from build123d import *

# Parameters (mm, degrees)
SKIZZE1_W                       = 100
SKIZZE1_H                       = 30
AUFSATZ_LINEAR_AUSTRAGEN1_DEPTH = 6
DURCHGANGSLOCH_F_R_M31_DEPTH    = 6
DURCHGANGSLOCH_F_R_M32_DEPTH    = 6
M3_GEWINDEBOHRUNG1_D            = 2.5
SKIZZE12_W                      = 12
SKIZZE12_H                      = 4
SCHNITT_LINEAR_AUSTRAGEN1_DEPTH = 25
VERRUNDUNG1_R                   = 2.5
SKIZZE13_W                      = 10
SKIZZE13_H                      = 30
SCHNITT_LINEAR_AUSTRAGEN2_DEPTH = 1.5
F_2_0MM_STIFTLOCH1_D            = 2
F_2_0MM_STIFTLOCH1_DEPTH        = 8.5
F_2_0MM_STIFTLOCH1_TIP          = 0.600860619


# Read off the part's stored shape, not the designer's step: Durchgangsloch für M31, Durchgangsloch für M32
with BuildPart() as part:
    # Skizze1 → Aufsatz-Linear austragen1 (new body)
    with BuildSketch(Plane(origin=(0, 0, 0), x_dir=(1, 0, 0), z_dir=(0, 1, 0))):
        Rectangle(SKIZZE1_W, SKIZZE1_H)
    extrude(amount=AUFSATZ_LINEAR_AUSTRAGEN1_DEPTH)

    # Durchgangsloch für M31 outline → Durchgangsloch für M31 (cut)
    with BuildSketch(Plane(origin=(0, 0, 0), x_dir=(1, 0, 0), z_dir=(0, 1, 0))):
        with BuildLine():
            Line((-43.4, -9.6), (23.4, -9.6))
            ThreePointArc((23.4, -9.6), (25, -8), (23.4, -6.4))
            Line((23.4, -6.4), (-43.4, -6.4))
            ThreePointArc((-43.4, -6.4), (-45, -8), (-43.4, -9.6))
        make_face()
        with BuildLine():
            Line((-43.4, 6.4), (23.4, 6.4))
            ThreePointArc((23.4, 6.4), (25, 8), (23.4, 9.6))
            Line((23.4, 9.6), (-43.4, 9.6))
            ThreePointArc((-43.4, 9.6), (-45, 8), (-43.4, 6.4))
        make_face()
    extrude(amount=DURCHGANGSLOCH_F_R_M31_DEPTH, mode=Mode.SUBTRACT)

    # Durchgangsloch für M32 outline → Durchgangsloch für M32 (cut)
    with BuildSketch(Plane(origin=(0, 0, 0), x_dir=(1, 0, 0), z_dir=(0, 1, 0))):
        with BuildLine():
            ThreePointArc((46.6, 10.605062793), (45, 12.205062793), (43.4, 10.605062793))
            Line((43.4, 10.605062793), (43.4, 3.805062793))
            ThreePointArc((43.4, 3.805062793), (45, 2.205062793), (46.6, 3.805062793))
            Line((46.6, 3.805062793), (46.6, 10.605062793))
        make_face()
        with BuildLine():
            Line((46.6, -10.605062793), (46.6, -3.805062793))
            ThreePointArc((46.6, -3.805062793), (45, -2.205062793), (43.4, -3.805062793))
            Line((43.4, -3.805062793), (43.4, -10.605062793))
            ThreePointArc((43.4, -10.605062793), (45, -12.205062793), (46.6, -10.605062793))
        make_face()
    extrude(amount=DURCHGANGSLOCH_F_R_M32_DEPTH, mode=Mode.SUBTRACT)

    # M3 Gewindebohrung1 (through all)
    with Locations(Plane(origin=(0, 6, 0), x_dir=(1, 0, 0), z_dir=(0, 1, 0))):
        with Locations((-40, 0), (-20, 0)):
            Hole(M3_GEWINDEBOHRUNG1_D / 2)

    # Skizze12 → Schnitt-Linear austragen1 (cut)
    with BuildSketch(Plane.ZY.offset(50)):
        with Locations((9, 2)):
            Rectangle(SKIZZE12_W, SKIZZE12_H)
    extrude(amount=-SCHNITT_LINEAR_AUSTRAGEN1_DEPTH, mode=Mode.SUBTRACT)

    # Verrundung1
    verrundung1_edges = [part.edges().sort_by_distance(p)[0] for p in [
        (-25, 2, 3),
    ]]
    fillet(verrundung1_edges, radius=VERRUNDUNG1_R)

    # Skizze13 → Schnitt-Linear austragen2 (cut)
    with BuildSketch(Plane(origin=(0, 6, 0), x_dir=(1, 0, 0), z_dir=(0, 1, 0))):
        with Locations((45, 0)):
            Rectangle(SKIZZE13_W, SKIZZE13_H)
    extrude(amount=-SCHNITT_LINEAR_AUSTRAGEN2_DEPTH, mode=Mode.SUBTRACT)

    # Ø2.0mm Stiftloch1
    with Locations(Plane(origin=(0, 4.5, 0), x_dir=(1, 0, 0), z_dir=(0, 1, 0))):
        with Locations((45, 0)):
            Hole(F_2_0MM_STIFTLOCH1_D / 2, depth=F_2_0MM_STIFTLOCH1_DEPTH)
            with Locations((0, 0, -(F_2_0MM_STIFTLOCH1_DEPTH + F_2_0MM_STIFTLOCH1_TIP / 2))):  # 118° drill point
                Cone(0, F_2_0MM_STIFTLOCH1_D / 2, F_2_0MM_STIFTLOCH1_TIP, mode=Mode.SUBTRACT)


solid = part.part
Read the model definition and answer for the solid it produces. Units are mm, in the model's axes. A direction names the side the tool comes from. Round coordinates to 2 decimals unless told otherwise and drop trailing zeros. Write each loop counter-clockwise with the first axis right and the second up, starting at its lowest first coordinate (ties: lowest second). Pieces come first, ordered by that corner, then holes.
1. The part is cut by section B-B, the plane x = 45. Determine the outline of the cut face in (y, z), then the cut area to 3 significant figures.
2. Straight lines are drawn through the part: L1, parallel to Z at x = -40, y = 2.55; L2, parallel to Z at x = -3.5, y = 2.45; L3, parallel to Z at x = -20, y = 3.5. For each, find the intervals that lie inside material, in ascending order.
3. Determine the mould class of faces 1 (the face through (45.035, 2.218, -12.205)), 2 (the face through (50, 2, 0)), 3 (the face through (43.8, 4.5, -0.2)) for opening direction X: pulls with the +X half, pulls with the -X half, needs draft (parallel to the pull), parting line crosses it, or undercut.
4. The part is cut by section C-C, the plane x = -36. Determine the outline of the cut face in (y, z), then the cut area to 3 significant figures.
5. Given pin 1 Ø3.5 at (x, z) = (-35.5, 10) entering from -Y; pin 2 Ø1 at (y, z) = (2.5, 6) entering from -X; pin 3 Ø3 at (x, y) = (-42.5, 2) entering from +Z, each flat-ended and moving along its own axis, determine where each tip first touches the part or whether it passes through.
6. The part is cut by section D-D, the plane x = -20. Determine the outline of the cut face in (y, z), then the cut area to 3 significant figures.
7. Which of the six approach directions +Z, -Z, +X, -X, +Y, -Y give full straight-line access (tool end or side, diameter ignored) to faces 4 (the face through (10, 3, 15)), 5 (the face through (-39, 2, 3)), 6 (the face through (-10, 3, -6.4))?
8. The part is cut by section A-A, the plane z = 8. Determine the outline of the cut face in (x, y), then the cut area to 3 significant figures.
Values:
1. outline: (0, -15) - (4.5, -15) - (4.5, -12.21) - (0, -12.21) - close; (0, -2.21) - (4.5, -2.21) - (4.5, -1) - (0, -1) - close; (0, 1) - (4.5, 1) - (4.5, 2.21) - (0, 2.21) - close; (0, 12.21) - (4.5, 12.21) - (4.5, 15) - (0, 15) - close
1. area: 36.0 mm2
2. L1: z = -15 to -9.6, -6.4 to -1.25, 1.25 to 3
2. L2: z = -15 to -9.6, -6.4 to 6.4, 9.6 to 15
2. L3: z = -15 to -9.6, -6.4 to -1.25, 1.25 to 6.4, 9.6 to 15
3. face 1: undercut
3. face 2: pulls with the +X half
3. face 3: needs draft
4. outline: (0, -15) - (6, -15) - (6, -9.6) - (0, -9.6) - close; (0, -6.4) - (6, -6.4) - (6, 6.4) - (4, 6.4) - (4, 3) - (0, 3) - close; (4, 9.6) - (6, 9.6) - (6, 15) - (4, 15) - close
4. area: 106 mm2
5. pin 1: stops at y = 4
5. pin 2: stops at x = -25
5. pin 3: stops at z = 3
6. outline: (0, -15) - (6, -15) - (6, -9.6) - (0, -9.6) - close; (0, -6.4) - (6, -6.4) - (6, -1.25) - (0, -1.25) - close; (0, 1.25) - (6, 1.25) - (6, 6.4) - (0, 6.4) - close; (0, 9.6) - (6, 9.6) - (6, 15) - (0, 15) - close
6. area: 127 mm2
7. face 4: +Z, +X, -X, +Y, -Y
7. face 5: +Z, -X, -Y
7. face 6: +Y, -Y
8. outline: (-50, 4) - (-45, 4) - (-45, 6) - (-50, 6) - close; (25, 0) - (43.4, 0) - (43.4, 4.5) - (40, 4.5) - (40, 6) - (25, 6) - close; (46.6, 0) - (50, 0) - (50, 4.5) - (46.6, 4.5) - close
8. area: 131 mm2
